Read the model definition and answer for the solid it produces. Units are mm, in the model's axes. A direction names the side the tool comes from. Give positions to 0.01 mm unless a question says otherwise; leave off trailing zeros. Loops run counter-clockwise (first coordinate to the right, second up) from the corner with the lowest first, then second, coordinate; pieces in that order, holes last. Notation, with made-up numbers: (4.5, 46) - (32.5, 46) arc R27 ccw to (32.5, 75) - close; hole circle Ø9 at (-10.75, 7.25). An arc over 180 degrees is marked (long way). Put each result on its own line as item: value. Start each with the question number.
1. A cutting plane is placed at A-A, the plane x = 0. Determine the outline of the cut face in (y, z).
2. Consider L1, parallel to X at y = 120.5, z = 7; L2, parallel to X at y = 41.5, z = 11; L3, parallel to Z at x = 6, y = 12. Determine where each line is inside the solid, lowest interval first. Write a range as from..to.
3. Given pin 1 Ø3 at (y, z) = (97, 7) entering from -X; pin 2 Ø8 at (x, y) = (9.5, 49.5) entering from +Z; pin 3 Ø3 at (x, y) = (12.5, 105.5) entering from +Z, each flat-ended and moving along its own axis, determine where each tip first touches the part or whether it passes through.
4. A cutting plane is placed at B-B, the plane y = 115. Determine the outline of the cut face in (x, z).
5. A cutting plane is placed at C-C, the plane z = 7. Determine the outline of the cut face in (x, y), plus the area to 3 significant figures.
6. A cutting plane is placed at D-D, the plane y = 54.5. Determine the outline of the cut face in (x, z).
7. For faces 1 (the flat face through (-8, 49, 24)), 2 (the flat face through (0, 0, -1)), determine the directions among +Z, -Z, +X, -X, +Y, -Y from which every point of the face is accessible in a straight line to the end or side of a thin tool.
8. For a pull along X with two mould halves and no side action, classify faces 3 (the flat face through (0, 150, 0)), 4 (the cylindrical face through (-27.334, 73.95, -6.07)), 5 (the flat face through (8, 49, 24)) as released by +X, released by -X, zero draft, split by the parting line, or undercut.
```python
from build123d import *

# Parameters (mm, degrees)
SKETCH1_R           = 28
BOSS_EXTRUDE1_DEPTH = 150
SKETCH2_W           = 16
SKETCH2_H           = 6
CUT_EXTRUDE1_DEPTH  = 100


with BuildPart() as part:
    # Sketch1 → Boss-Extrude1 (new body)
    with BuildSketch(Plane(origin=(0, 0, 0), x_dir=(1, 0, 0), z_dir=(0, 1, 0))):
        with Locations(Location((0, 0, 0), (0, 0, 270))):
            Circle(SKETCH1_R)
    extrude(amount=BOSS_EXTRUDE1_DEPTH)

    # Sketch2 → Cut-Extrude1 (cut)
    with BuildSketch(Plane.XZ):
        with Locations((0, 25)):
            Rectangle(SKETCH2_W, SKETCH2_H)
    extrude(amount=-CUT_EXTRUDE1_DEPTH, mode=Mode.SUBTRACT)


solid = part.part
```
Return value:
1. outline: (0, -28) - (150, -28) - (150, 28) - (100, 28) - (100, 22) - (0, 22) - close
2. L1: x = -27.11..27.11
2. L2: x = -25.75..25.75
2. L3: z = -27.35..22
3. pin 1: stops at x = -27.45
3. pin 2: stops at z = 26.83
3. pin 3: stops at z = 25.75
4. outline: circle Ø56 at (0, 0)
5. outline: (-27.11, 0) - (27.11, 0) - (27.11, 150) - (-27.11, 150) - close
5. area: 8,130 mm2
6. outline: (-8, 22) - (-8, 26.83) arc R28 ccw (long way) to (8, 26.83) - (8, 22) - close
7. face 1: +Z, -Y
7. face 2: +Z, -Z, +X, -X, -Y
8. face 3: zero draft
8. face 4: split by the parting line
8. face 5: undercut
